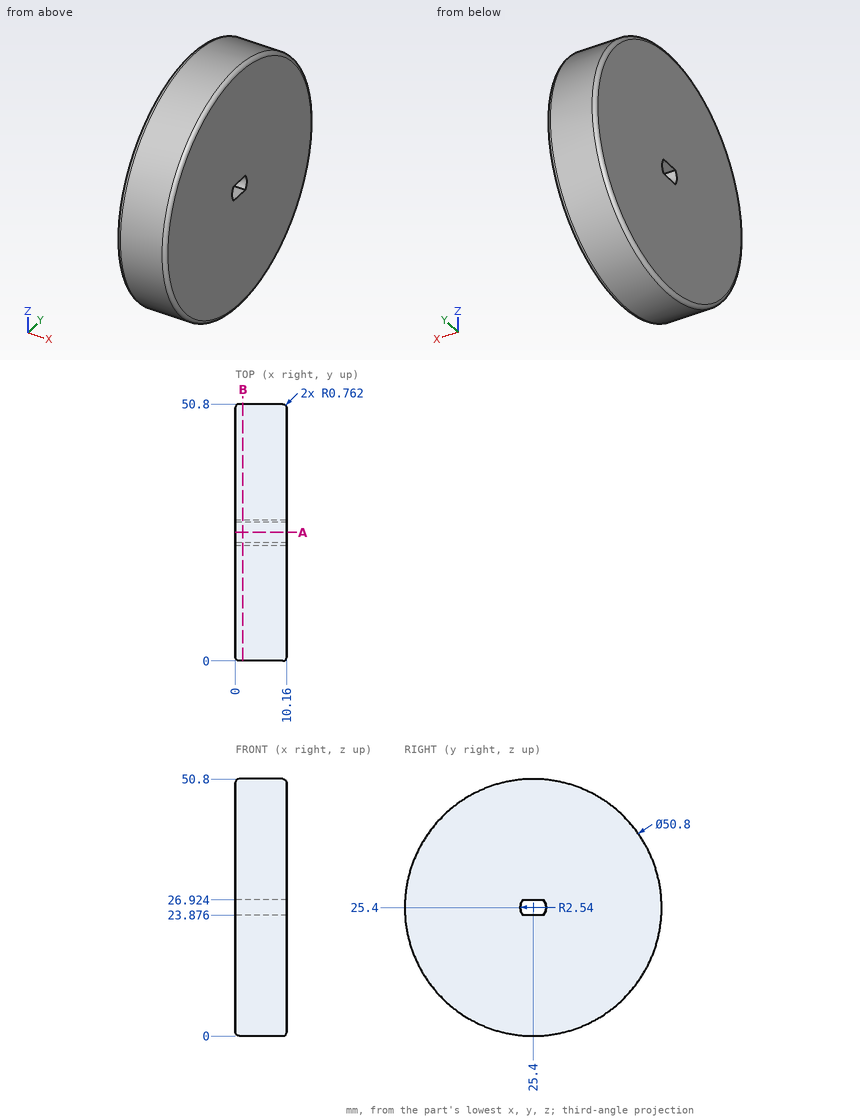
Print and shaded views of the part. All mm, measured from the part's lowest x, y and z. Round coordinates to 2 decimals unless told otherwise and drop trailing zeros. Write each loop counter-clockwise with the first axis right and the second up, starting at its lowest first coordinate (ties: lowest second). Pieces come first, ordered by that corner, then holes. Notation, with made-up numbers: (-17.5, 46) -> (28.5, 46) arc R25 ccw to (28.5, 73) -> close; hole circle Ø4 at (-35.75, -7). An arc over 180 degrees is marked (long way). Return JSON: item names as keys, results as strings. Group by question number.
Q1. Saw through at A-A on y = 25.4. Write the cut outline in (x, z), plus the area to 3 significant figures.
Q2. Pin check, flat tips, straight feed: pin 1 (2 mm diameter, centred on x = 7, y = 26, fed in from +Z); pin 2 (1 mm diameter, centred on x = 6.5, z = 13, fed in from +Y); pin 3 (5 mm diameter, centred on x = 7.5, y = 5.5, fed in from +Z); pin 4 (2 mm diameter, centred on x = 7, z = 17, fed in from -Y). Stop position of each tip, or through.
Q3. Probe L1, parallel to Z at x = 5.5, y = 24; L2, parallel to Y at x = 3.5, z = 48.5; L3, parallel to Z at x = 3.25, y = 10. List the from-to ranges inside material, lowest first. Write a range as [from, to].
Q4. Saw through at B-B on x = 1.5. Write the cut outline in (y, z).
Answer:
{
 "1": {"outline": "(0, 0.76) arc R0.76 ccw to (0.76, 0) -> (9.4, 0) arc R0.76 ccw to (10.16, 0.76) -> (10.16, 23.88) -> (0, 23.88) -> close; (0, 26.92) -> (10.16, 26.92) -> (10.16, 50.04) arc R0.76 ccw to (9.4, 50.8) -> (0.76, 50.8) arc R0.76 ccw to (0, 50.04) -> close", "area": "485 mm2"},
 "2": {"pin 1": "z = 50.8", "pin 2": "y = 47.84", "pin 3": "z = 43.9", "pin 4": "y = 1.1"},
 "3": {"L1": "[0.04, 23.88], [26.92, 50.76]", "L2": "[14.84, 35.96]", "L3": "[5.2, 45.6]"},
 "4": {"outline": "circle Ø50.8 at (25.4, 25.4); hole (23.37, 23.88) -> (27.43, 23.88) arc R2.54 ccw to (27.43, 26.92) -> (23.37, 26.92) arc R2.54 ccw to start"}
}
